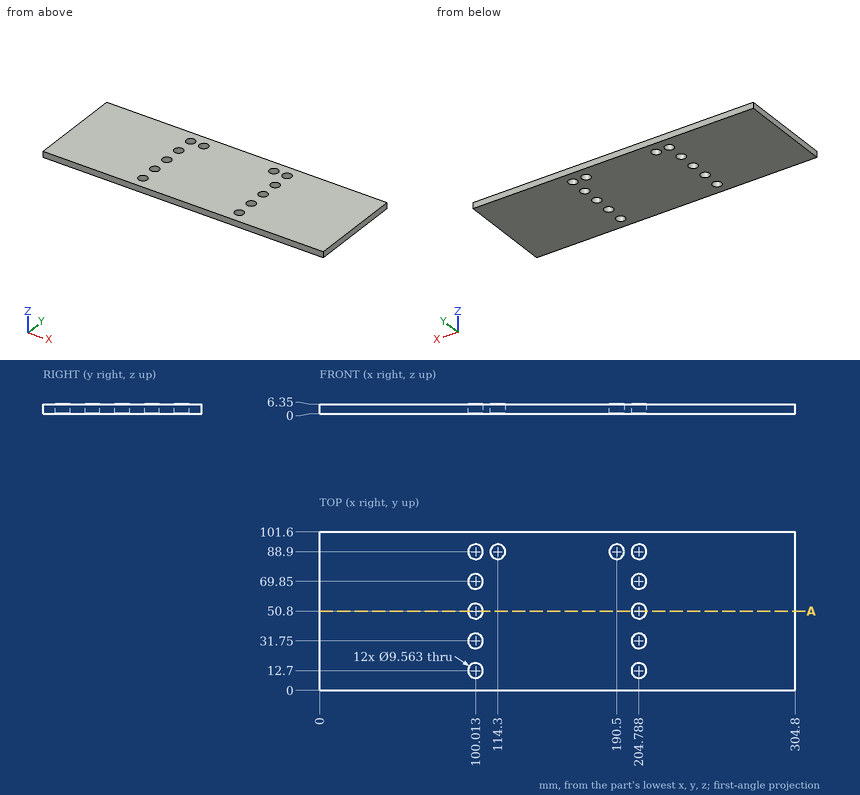
Print and shaded views of the part. All mm, measured from the part's lowest x, y and z. Round coordinates to 2 decimals unless told otherwise and drop trailing zeros.
Item 1: Drop flat-ended pins along their axis: pin 1 Ø15.5 at (x, y) = (204.79, 12.7) entering from +Z; pin 2 Ø5.5 at (x, y) = (100.01, 31.75) entering from -Z. Give the stop position or say it passes through.
Results:
pin 1: stops at z = 6.35
pin 2: passes through
Item 2: Probe L1, parallel to X at y = 28.5, z = 3.5 (1 decimal); L2, parallel to X at y = 17, z = 0.5 (1 decimal). List the from-to ranges inside material, lowest first.
Results:
L1: x = 0 to 96.5, 103.5 to 201.3, 208.3 to 304.8
L2: x = 0 to 97.9, 102.1 to 202.7, 206.9 to 304.8
Item 3: Cut at A-A, the plane y = 50.8. Count the separate pieces of the cut face and the enclosed holes in it, plus the area to 3 significant figures.
Results:
separate pieces: 3
enclosed holes: 0
area: 1,810 mm2
